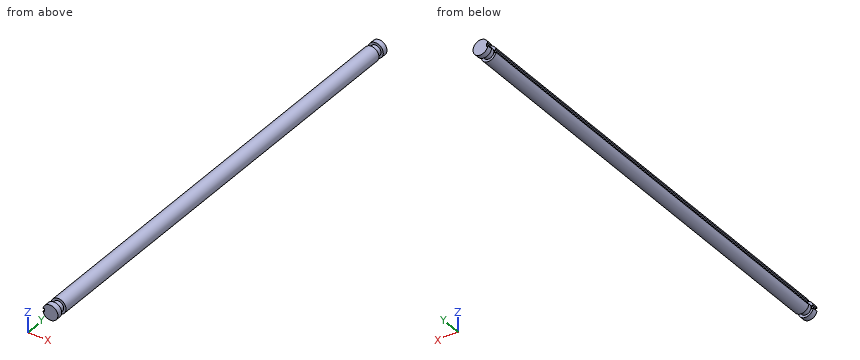
```python
from build123d import *

# Parameters (mm, degrees)
CUT_EXTRUDE2_START = -998.728
SKETCH2_W          = 63.4619
SKETCH2_H          = 12.7
CUT_EXTRUDE2_DEPTH = 1997.456


with BuildPart() as part:
    # Sketch1 → Revolve1 (revolve)
    with BuildSketch(Plane(origin=(0, 0, 0), x_dir=(0, 1, 0), z_dir=(0, 0, 1)), mode=Mode.PRIVATE) as revolve1_sk:
        Polygon((-976.376, 0), (-976.376, 31.73095), (-954.024, 31.73095), (-954.024, 22.0218), (-928.2176, 22.0218), (-928.2176, 31.73095), (928.3446, 31.73095), (928.3446, 22.0218), (954.151, 22.0218), (954.151, 31.73095), (976.376, 31.73095), (976.376, 0), align=None)
    revolve(revolve1_sk.sketch.rotate(Axis((0, -1001.776, 0), (0, 1, 0)), 270), axis=Axis((0, -1001.776, 0), (0, 1, 0)))

    # Sketch2 → Cut-Extrude2 (cut)
    with BuildSketch(Plane(origin=(0, 0, 0), x_dir=(-1, 0, 0), z_dir=(0, 1, 0)).offset(CUT_EXTRUDE2_START)):
        with Locations((56.3372, 0)):
            Rectangle(SKETCH2_W, SKETCH2_H)
    extrude(amount=CUT_EXTRUDE2_DEPTH, mode=Mode.SUBTRACT)


solid = part.part
```
Could you check a few things on this model? Use its own coordinates, in mm. Coordinates: 2 decimals unless noted, no trailing zeros. Loops run counter-clockwise (first coordinate to the right, second up) from the corner with the lowest first, then second, coordinate; pieces in that order, holes last. Notation, with made-up numbers: M 25,7 L 67,7 A31 ccw 67,39 Z; hole C 44,54 d7. An arc over 180 degrees is marked long. Put each result on its own line as item: value. Start each with the question number.
(1) I need wall thicknesses on line 1 (Y direction, x = 16.5, z = 26.5); line 2 (X direction, y = -807.5, z = 23); line 3 (Z direction, x = -22.5, y = -640). Which ranges of each line are inside material? Lowest first, please. Write a range as from..to.
(2) Suppose I cut it at A-A on y = -553.5. Please give me the cut outline in (x, z), then the cut area to 3 significant figures.
(3) Suppose I cut it at B-B on x = -10. Please give me the cut outline in (y, z).
(4) Will these pins go through, and if not, where does the flat tip stop? P1, Ø6, axis at x = 5, y = 742, coming from the -Z side; P2, Ø5, axis at x = -29, y = -142.5, coming from the +Z side; P3, Ø10, axis at y = -326, z = -2.5, coming from the -X side.
Solutions:
1. line 1: y = -976.38..-954.02, -928.22..928.34, 954.15..976.38
1. line 2: x = -21.86..21.86
1. line 3: z = -22.37..22.37
2. outline: M -31.09,-6.35 A31.73 ccw long -31.09,6.35 L -24.61,6.35 L -24.61,-6.35 Z
2. area: 3,080 mm2
3. outline: M -976.38,-30.11 L -954.02,-30.11 L -954.02,-19.62 L -928.22,-19.62 L -928.22,-30.11 L 928.34,-30.11 L 928.34,-19.62 L 954.15,-19.62 L 954.15,-30.11 L 976.38,-30.11 L 976.38,30.11 L 954.15,30.11 L 954.15,19.62 L 928.34,19.62 L 928.34,30.11 L -928.22,30.11 L -928.22,19.62 L -954.02,19.62 L -954.02,30.11 L -976.38,30.11 Z
4. P1: stops at z = -31.67
4. P2: stops at z = 17.45
4. P3: stops at x = -31.09
